Geometry: final body of the model. Coordinates: model frame, mm. A direction names the side the tool comes from. Give positions to 0.01 mm unless a question says otherwise; leave off trailing zeros. Loops run counter-clockwise (first coordinate to the right, second up) from the corner with the lowest first, then second, coordinate; pieces in that order, holes last. Notation, with made-up numbers: (72.5, 21.25) - (88.5, 21.25) arc R25 ccw to (88.5, 53.25) - close; hole circle Ø2 at (-21.75, 55.25). An arc over 180 degrees is marked (long way). Answer in a Markdown table with one row per item.
Autodesk Inventor part; units mm, degrees
ref_plane "YZ Plane" through (0, 0, 0) normal (1, 0, 0) x (0, 1, 0)
ref_plane "XZ Plane" through (0, 0, 0) normal (0, 1, 0) x (-1, 0, 0)
ref_plane "XY Plane" through (0, 0, 0) normal (0, 0, 1) x (1, 0, 0)
sketch "Sketch1" plane through (0, 0, 0) normal (0, 0, 1) x (1, 0, 0)
  line L0 (0, 0) -> (76.2, 0)
  line L1 (76.2, 0) -> (76.2, 25.4)
  line L2 (76.2, 25.4) -> (25.4, 25.4)
  line L3 (0, 25.4) -> (0, 0)
  line L4 (0, 0) -> (25.4, 0)
  line L5 (25.4, 25.4) -> (25.4, 76.2)
  line L6 (25.4, 76.2) -> (0, 76.2)
  line L7 (0, 76.2) -> (0, 0)
  line L8 (12.7, 76.2) -> (12.7, 63.5) construction
  line L9 (12.7, 63.5) -> (12.7, 38.1) construction
  line L10 (12.7, 38.1) -> (12.7, 12.7) construction
  line L11 (12.7, 12.7) -> (38.1, 12.7) construction
  line L12 (38.1, 12.7) -> (63.5, 12.7) construction
  circle A0 centre (12.7, 63.5) radius 2.5797
  circle A1 centre (12.7, 38.1) radius 2.5797
  circle A2 centre (12.7, 12.7) radius 2.5797
  circle A3 centre (38.1, 12.7) radius 2.5797
  circle A4 centre (63.5, 12.7) radius 2.5797
  dimension "d0" = 76.2
  dimension "d1" = 25.4
  dimension "d2" = 25.4
  dimension "d3" = 76.2
  dimension "d4" = 12.7
  dimension "d5" = 25.4
  dimension "d6" = 25.4
  dimension "d7" = 25.4
  dimension "d8" = 25.4
  dimension "d9" = 5.1594
extrude "Extrusion1" add sketch "Sketch1" along normal blind 3.175
sketch "Sketch2" plane through (0, 0, 3.175) normal (0, 0, 1) x (1, 0, 0)
  line L0 (0, 0) -> (76.2, 0) construction
  line L1 (0, 0) -> (9.7028, 0) construction
  line L2 (9.7028, 0) -> (9.7028, 6.5024) construction
  circle A0 centre (9.7028, 6.5024) radius 3.302
  dimension "d12" = 9.7028
  dimension "d13" = 6.5024
  dimension "d14" = 6.604
extrude "Extrusion2" cut sketch "Sketch2" against normal blind 25.4
properties part number "L gusset"
Q1. First-contact query: pin 1 (6 mm diameter, centred on x = 9.7, y = 6.5, fed in from -Z). Flat tip, straight axial feed; report the tip coordinate or a pass-through.
Check values:
| item | result |
|---|---|
| pin 1 | through |
Q2. Cut plane A-A (y = 38.1). Output: boundary loops of the cut face in (x, z) (3 decimals).
Check values:
| item | result |
|---|---|
| outline | (0, 0) - (10.12, 0) - (10.12, 3.175) - (0, 3.175) - close; (15.28, 0) - (25.4, 0) - (25.4, 3.175) - (15.28, 3.175) - close |
Q3. Material intervals for line 1 along X through (y, z) = (12.5, 2.05); line 2 along Y through (x, z) = (12.7, 1.85); line 3 along Y through (x, z) = (63.5, 1.45), sorted ascending.
Check values:
| item | result |
|---|---|
| line 1 | 0 to 10.13, 15.27 to 35.53, 40.67 to 60.93, 66.07 to 76.2 |
| line 2 | 0 to 5.12, 7.89 to 10.12, 15.28 to 35.52, 40.68 to 60.92, 66.08 to 76.2 |
| line 3 | 0 to 10.12, 15.28 to 25.4 |
Q4. Cut plane B-B (y = 12.7). Output: boundary loops of the cut face in (x, z) (3 decimals).
Check values:
| item | result |
|---|---|
| outline | (0, 0) - (10.12, 0) - (10.12, 3.175) - (0, 3.175) - close; (15.28, 0) - (35.52, 0) - (35.52, 3.175) - (15.28, 3.175) - close; (40.68, 0) - (60.92, 0) - (60.92, 3.175) - (40.68, 3.175) - close; (66.08, 0) - (76.2, 0) - (76.2, 3.175) - (66.08, 3.175) - close |
Q5. Cut plane C-C (z = 2.65). Output: boundary loops of the cut face in (x, y).
Check values:
| item | result |
|---|---|
| outline | (0, 0) - (76.2, 0) - (76.2, 25.4) - (25.4, 25.4) - (25.4, 76.2) - (0, 76.2) - close; hole circle Ø6.6 at (9.7, 6.5); hole circle Ø5.16 at (12.7, 12.7); hole circle Ø5.16 at (12.7, 38.1); hole circle Ø5.16 at (12.7, 63.5); hole circle Ø5.16 at (38.1, 12.7); hole circle Ø5.16 at (63.5, 12.7) |
Q6. Reachability of faces 1 (the flat face through (38, 0, 2)), 2 (the flat face through (25.4, 50, 2)) from +Z, -Z, +X, -X, +Y, -Y: full face, straight path, thin tool, end or side. Return the list, or none.
Check values:
| item | result |
|---|---|
| face 1 | +Z, -Z, +X, -X, -Y |
| face 2 | +Z, -Z, +X, +Y |
Q7. Draft query along X for faces 3 (the flat face through (21, 30, 3.175)), 4 (the flat face through (76.2, 13, 2)), 5 (the cylindrical face through (7.269, 8.734, 1.61)). Return one class per face: pulls with the +X half, pulls with the -X half, needs draft (parallel to the pull), parting line crosses it, or undercut.
Check values:
| item | result |
|---|---|
| face 3 | needs draft |
| face 4 | pulls with the +X half |
| face 5 | undercut |
Q8. Cut plane D-D (x = 70.5). Output: boundary loops of the cut face in (y, z) (3 decimals), and give its area (3 significant figures).
Check values:
| item | result |
|---|---|
| outline | (0, 0) - (25.4, 0) - (25.4, 3.175) - (0, 3.175) - close |
| area | 80.6 mm² |
